Work out the finished part from the listing and answer in its coordinate system (mm). A direction names the side the tool comes from. Coordinates: 2 decimals unless noted, no trailing zeros. Loops run counter-clockwise (first coordinate to the right, second up) from the corner with the lowest first, then second, coordinate; pieces in that order, holes last. Notation, with made-up numbers: (-28.75, 83.5) -> (14.25, 83.5) arc R32 ccw to (14.25, 114.5) -> close; hole circle Ø5 at (65, -22). An arc over 180 degrees is marked (long way). One line per question, with ' | ' between items.
```python
from build123d import *

# Parameters (mm, degrees)
BOSS_EXTRUDE1_DEPTH     = 5
SKETCH3_R               = 1.6
CUT_EXTRUDE1_DEPTH      = 1
CUT_EXTRUDE1_DEPTH_BACK = 6
SKETCH4_R               = 2.55
CUT_EXTRUDE2_DEPTH      = 10
SKETCH5_R               = 1.55
CUT_EXTRUDE3_DEPTH      = 6
SKETCH6_R               = 1.55
CUT_EXTRUDE4_DEPTH      = 6
SKETCH7_W               = 23
SKETCH7_H               = 110
BOSS_EXTRUDE2_DEPTH     = 5
SKETCH9_W               = 5
SKETCH9_H               = 40
BOSS_EXTRUDE4_DEPTH     = 33
SKETCH11_W              = 12
SKETCH11_H              = 12
CUT_EXTRUDE5_DEPTH      = 50
SKETCH12_R              = 1.6
CUT_EXTRUDE6_DEPTH      = 50
SKETCH13_W              = 15
SKETCH13_H              = 15
SKETCH13_R              = 1.6
BOSS_EXTRUDE5_DEPTH     = 14.25
SKETCH15_W              = 89.5
SKETCH15_H              = 3.65
CUT_EXTRUDE9_DEPTH      = 111
SKETCH18_W              = 13
SKETCH18_H              = 110
CUT_EXTRUDE10_DEPTH     = 6
FILLET5_R               = 5
SKETCH19_R              = 1.55
CUT_EXTRUDE11_DEPTH     = 5


with BuildPart() as part:
    # Sketch1 → Boss-Extrude1 (new body)
    with BuildSketch(Plane(origin=(0, 0, 0), x_dir=(1, 0, 0), z_dir=(0, 1, 0))):
        Polygon((75, 85), (-75, 85), (-75, -25), (-45, -45), (-45, -80), (45, -80), (45, -45), (75, -25), align=None)
        Polygon((-18.5, -10), (-18.5, 10), (-7.5, 10), (-7.5, 50), (7.5, 50), (7.5, 10), (18.5, 10), (18.5, -10), align=None, mode=Mode.SUBTRACT)
    extrude(amount=BOSS_EXTRUDE1_DEPTH)

    # Sketch3 → Cut-Extrude1 (cut, two sides)
    with BuildSketch(Plane(origin=(0, 5, 0), x_dir=(1, 0, 0), z_dir=(0, 1, 0))) as cut_extrude1_sk:
        with Locations((-35, 20)):
            Circle(SKETCH3_R)
        with Locations((-35, -20)):
            Circle(SKETCH3_R)
        with Locations((35, -20)):
            Circle(SKETCH3_R)
        with Locations((35, 20)):
            Circle(SKETCH3_R)
    extrude(amount=CUT_EXTRUDE1_DEPTH, mode=Mode.SUBTRACT)
    extrude(cut_extrude1_sk.sketch, amount=-CUT_EXTRUDE1_DEPTH_BACK, mode=Mode.SUBTRACT)

    # Sketch4 → Cut-Extrude2 (cut)
    with BuildSketch(Plane(origin=(0, 5, 0), x_dir=(1, 0, 0), z_dir=(0, 1, 0))):
        with Locations((-65, 66)):
            Circle(SKETCH4_R)
        with Locations((65, -4)):
            Circle(SKETCH4_R)
        with Locations((-65, -4)):
            Circle(SKETCH4_R)
        with Locations((65, 66)):
            Circle(SKETCH4_R)
    extrude(amount=-CUT_EXTRUDE2_DEPTH, mode=Mode.SUBTRACT)

    # Sketch5 → Cut-Extrude3 (cut, through all)
    with BuildSketch(Plane(origin=(0, 5, 0), x_dir=(1, 0, 0), z_dir=(0, 1, 0))):
        with Locations((-39, -75)):
            Circle(SKETCH5_R)
        with Locations((39, -75)):
            Circle(SKETCH5_R)
        with Locations((-39, -50)):
            Circle(SKETCH5_R)
        with Locations((39, -50)):
            Circle(SKETCH5_R)
    extrude(amount=-CUT_EXTRUDE3_DEPTH, mode=Mode.SUBTRACT)

    # Sketch6 → Cut-Extrude4 (cut, through all)
    with BuildSketch(Plane(origin=(0, 5, 0), x_dir=(1, 0, 0), z_dir=(0, 1, 0))):
        with Locations((62.5, 80)):
            Circle(SKETCH6_R)
        with Locations((-62.5, 80)):
            Circle(SKETCH6_R)
    extrude(amount=-CUT_EXTRUDE4_DEPTH, mode=Mode.SUBTRACT)

    # Sketch7 → Boss-Extrude2 (add)
    with BuildSketch(Plane(origin=(0, 5, 0), x_dir=(1, 0, 0), z_dir=(0, 1, 0))):
        with Locations((-86.5, 30)):
            Rectangle(SKETCH7_W, SKETCH7_H)
        with Locations((86.5, 30)):
            Rectangle(SKETCH7_W, SKETCH7_H)
    extrude(amount=-BOSS_EXTRUDE2_DEPTH)

    # Sketch9 → Boss-Extrude4 (add)
    with BuildSketch(Plane(origin=(0, 5, 0), x_dir=(1, 0, 0), z_dir=(0, 1, 0))):
        with Locations((-42.25, -5)):
            Rectangle(SKETCH9_W, SKETCH9_H)
        with Locations((42.25, -5)):
            Rectangle(SKETCH9_W, SKETCH9_H)
    extrude(amount=BOSS_EXTRUDE4_DEPTH)

    # Sketch11 → Cut-Extrude5 (cut)
    with BuildSketch(Plane(origin=(0, 5, 0), x_dir=(1, 0, 0), z_dir=(0, 1, 0))):
        with Locations((-67, 18.305755671)):
            Rectangle(SKETCH11_W, SKETCH11_H)
        with Locations((67, 18.305755671)):
            Rectangle(SKETCH11_W, SKETCH11_H)
    extrude(amount=-CUT_EXTRUDE5_DEPTH, mode=Mode.SUBTRACT)

    # Sketch12 → Cut-Extrude6 (cut)
    with BuildSketch(Plane.ZY.offset(44.75)):
        with Locations((0, 31.85)):
            Circle(SKETCH12_R)
        with Locations((5, 26.85)):
            Circle(SKETCH12_R)
        with Locations((0, 21.85)):
            Circle(SKETCH12_R)
        with Locations((-5, 26.85)):
            Circle(SKETCH12_R)
    cut_extrude6 = extrude(amount=-CUT_EXTRUDE6_DEPTH, mode=Mode.SUBTRACT)

    # Sketch13 → Boss-Extrude5 (add)
    with BuildSketch(Plane.ZY.offset(44.75)):
        with Locations((0, 26.85)):
            Rectangle(SKETCH13_W, SKETCH13_H)
        with Locations((0, 31.85)):
            Circle(SKETCH13_R, mode=Mode.SUBTRACT)
        with Locations((5, 26.85)):
            Circle(SKETCH13_R, mode=Mode.SUBTRACT)
        with Locations((-5, 26.85)):
            Circle(SKETCH13_R, mode=Mode.SUBTRACT)
        with Locations((0, 21.85)):
            Circle(SKETCH13_R, mode=Mode.SUBTRACT)
    boss_extrude5 = extrude(amount=BOSS_EXTRUDE5_DEPTH)

    # Mirror2: Cut-Extrude6 across plane
    add(cut_extrude6.mirror(Plane.ZY), mode=Mode.SUBTRACT)

    # Mirror3: Boss-Extrude5 across plane
    add(boss_extrude5.mirror(Plane.ZY))

    # Sketch15 → Cut-Extrude9 (cut, through all)
    with BuildSketch(Plane.XY.offset(25)):
        with Locations((0, 36.175)):
            Rectangle(SKETCH15_W, SKETCH15_H)
    extrude(amount=-CUT_EXTRUDE9_DEPTH, mode=Mode.SUBTRACT)

    # Sketch18 → Cut-Extrude10 (cut, through all)
    with BuildSketch(Plane(origin=(0, 5, 0), x_dir=(1, 0, 0), z_dir=(0, 1, 0))):
        with Locations((-91.5, 30)):
            Rectangle(SKETCH18_W, SKETCH18_H)
        with Locations((91.5, 30)):
            Rectangle(SKETCH18_W, SKETCH18_H)
    extrude(amount=-CUT_EXTRUDE10_DEPTH, mode=Mode.SUBTRACT)

    # Fillet5
    fillet5_edges = [part.edges().sort_by_distance(p)[0] for p in [
        (-44.75, 19.35, 0),
        (44.75, 19.35, 0),
    ]]
    fillet(fillet5_edges, radius=FILLET5_R)

    # Sketch19 → Cut-Extrude11 (cut)
    with BuildSketch(Plane(origin=(0, 5, 0), x_dir=(1, 0, 0), z_dir=(0, 1, 0))):
        with Locations((55, 34.5)):
            Circle(SKETCH19_R)
        with Locations((25, 34.5)):
            Circle(SKETCH19_R)
        with Locations((25, 44.5)):
            Circle(SKETCH19_R)
        with Locations((55, 44.5)):
            Circle(SKETCH19_R)
    cut_extrude11 = extrude(amount=-CUT_EXTRUDE11_DEPTH, mode=Mode.SUBTRACT)

    # Mirror4: Cut-Extrude11 across plane
    add(cut_extrude11.mirror(Plane.ZY), mode=Mode.SUBTRACT)


solid = part.part
```
1) Find section A-A (x = 10). Write down the section's boundary in (y, z).
Check values:
outline: (0, -85) -> (5, -85) -> (5, -10) -> (0, -10) -> close; (0, 10) -> (5, 10) -> (5, 80) -> (0, 80) -> close
2) Find the intervals of material crossed by line 1 along Z through (x, y) = (54.75, 26.85); line 2 along Z through (x, y) = (-25, 1.7); line 3 along X through (y, z) = (4, 75), in increasing order.
Check values:
line 1: z = -7.5 to -6.6, -3.4 to 3.4, 6.6 to 7.5 | line 2: z = -85 to -46.05, -42.95 to -36.05, -32.95 to 80 | line 3: x = -45 to -40.55, -37.45 to 37.45, 40.55 to 45
3) The mould has two halves that part along X. Classify faces 1 (the face through (60, 2, 35)), 2 (the face through (0, 2, 10)), 3 (the face through (-80, 3, 25)): released by +X, released by -X, zero draft, split by the parting line, or undercut.
Check values:
face 1: released by +X | face 2: undercut | face 3: zero draft
4) For faces 4 (the face through (-42, 19, -15)), 5 (the face through (0, 2, -50)), 6 (the face through (52, 26, 7.5)), determine the directions among +Z, -Z, +X, -X, +Y, -Y from which every point of the face is accessible in a straight line to the end or side of a thin tool.
Check values:
face 4: -Z, +X, -X, +Y | face 5: +Y, -Y | face 6: +Z, +X, +Y
5) Find section D-D (z = 57.5). Write down the section's boundary in (x, y).
Check values:
outline: (-45, 0) -> (45, 0) -> (45, 5) -> (-45, 5) -> close
6) Find section C-C (z = -58.5). Write down the section's boundary in (x, y).
Check values:
outline: (-85, 0) -> (85, 0) -> (85, 5) -> (-85, 5) -> close
7) Flat-ended cylindrical pins translate along their axes: pin 1 (10 mm diameter, centred on x = -21.5, z = 30, fed in from +Y); pin 2 (3 mm diameter, centred on x = 38.5, y = 13, fed in from -Z); pin 3 (2.5 mm diameter, centred on x = 55, z = -44.5, fed in from -Y); pin 4 (12 mm diameter, centred on y = 19.5, z = -17, fed in from -X). Find the tip coordinate at first contact, or state that the pin passes through.
Check values:
pin 1: stops at y = 5 | pin 2: stops at z = -15 | pin 3: passes through | pin 4: stops at x = -44.75
8) Find section B-B (y = 10). Write down the section's boundary in (x, z).
Check values:
outline: (-44.75, -15) -> (-39.75, -15) -> (-39.75, 25) -> (-44.75, 25) -> close; (39.75, -15) -> (44.75, -15) -> (44.75, 25) -> (39.75, 25) -> close
